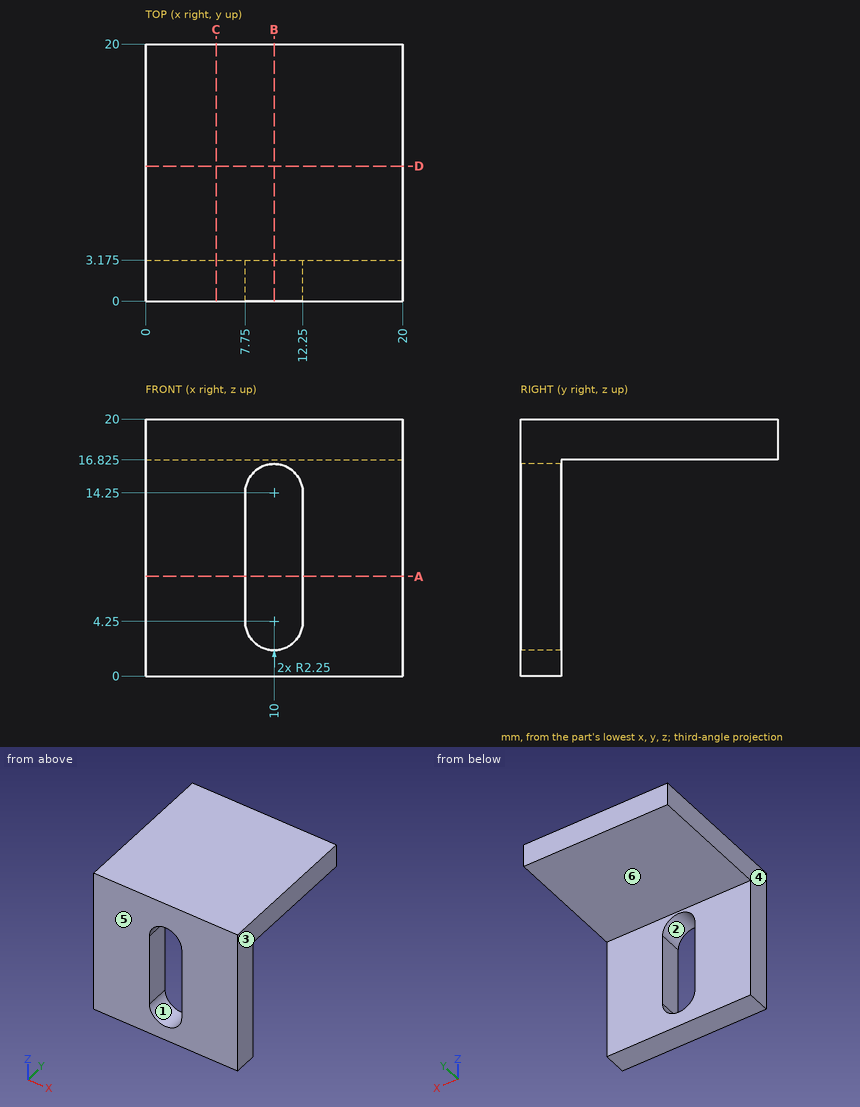
Check sheet for the drawn part. Datum: minimum x, y, z corner. Units: mm. A direction names the side the tool comes from. Give positions to 0.01 mm unless a question says otherwise; leave off trailing zeros. Order: outer loops, then holes, each group sorted by start corner. A loop starts at its lowest first (then second) coordinate and runs counter-clockwise, first axis right, second up.
1. Scan lines: line 1 (X direction, y = 2, z = 8.25); line 2 (Y direction, x = 3, z = 2.5) (3 decimals); line 3 (Z direction, x = 5.25, y = 13) (3 decimals). Record each from-to range of solid material in increasing order.
Completed:
line 1: x = 0 to 7.75, 12.25 to 20
line 2: y = 0 to 3.175
line 3: z = 16.825 to 20
2. Depth check by flat-ended pin: pin 1 (3 mm diameter, centred on x = 9.5, y = 12.5, fed in from -Z) (3 decimals); pin 2 (10 mm diameter, centred on x = 4, z = 11, fed in from +Y) (3 decimals); pin 3 (6 mm diameter, centred on y = 8.5, z = 4.5, fed in from +X). Enter the tip coordinate at first touch or a pass-through.
Completed:
pin 1: stops at z = 16.825
pin 2: stops at y = 3.175
pin 3: passes through
3. Access from +Z, -Z, +X, -X, +Y, -Y to the whole of each face (thin tool, end or side, straight path). Record for the marked faces 5 and 6.
Completed:
face 5: +Z, -Z, +X, -X, -Y
face 6: -Z, +X, -X, +Y
4. Draft check along X on the marked faces 1, 2, 3 and 4. Enter one of: pulls with the +X half, pulls with the -X half, needs draft (parallel to the pull), parting line crosses it, or undercut.
Completed:
face 1: undercut
face 2: undercut
face 3: pulls with the +X half
face 4: pulls with the -X half
5. Sectioned sample at B-B (x = 10). Record the boundary of the cut face in (y, z) (3 decimals).
Completed:
outline: (0, 0) - (3.175, 0) - (3.175, 2) - (0, 2) - close; (0, 16.5) - (3.175, 16.5) - (3.175, 16.825) - (20, 16.825) - (20, 20) - (0, 20) - close
6. Sectioned sample at A-A (z = 7.75). Record the boundary of the cut face in (x, y) (3 decimals), then the cut area to 3 significant figures.
Completed:
outline: (0, 0) - (7.75, 0) - (7.75, 3.175) - (0, 3.175) - close; (12.25, 0) - (20, 0) - (20, 3.175) - (12.25, 3.175) - close
area: 49.2 mm2
7. Sectioned sample at C-C (x = 5.5). Record the boundary of the cut face in (y, z) (3 decimals), then the cut area to 3 significant figures.
Completed:
outline: (0, 0) - (3.175, 0) - (3.175, 16.825) - (20, 16.825) - (20, 20) - (0, 20) - close
area: 117 mm2
8. Sectioned sample at D-D (y = 10.5). Record the boundary of the cut face in (x, z) (3 decimals), then the cut area to 3 significant figures.
Completed:
outline: (0, 16.825) - (20, 16.825) - (20, 20) - (0, 20) - close
area: 63.5 mm2
